Could you check a few things on this drawing? It's one solid part, dimensions in mm from its lowest x, y, z. A direction names the side the tool comes from. Coordinates: 2 decimals unless noted, no trailing zeros. Loops run counter-clockwise (first coordinate to the right, second up) from the corner with the lowest first, then second, coordinate; pieces in that order, holes last. Notation, with made-up numbers: (66.5, 50.25) -> (93.5, 50.25) arc R22 cw to (93.5, 88.25) -> close; hole circle Ø9 at (87, 1.25). An arc over 180 degrees is marked (long way). One line per question, with ' | ' between items.
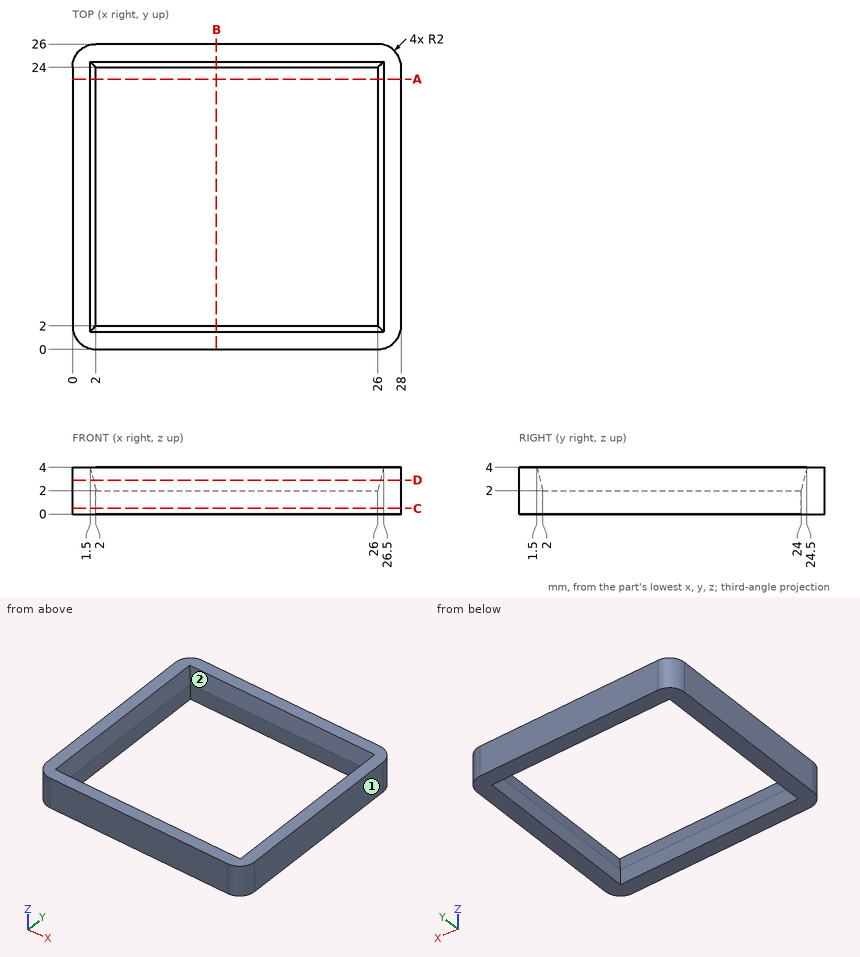
1) If we section it at D-D on z = 2.9: Please give me the cut outline in (x, y) (3 decimals), and give its area (3 significant figures).
Data:
outline: (0, 2) arc R2 ccw to (2, 0) -> (26, 0) arc R2 ccw to (28, 2) -> (28, 24) arc R2 ccw to (26, 26) -> (2, 26) arc R2 ccw to (0, 24) -> close; hole (1.775, 1.775) -> (26.225, 1.775) -> (26.225, 24.225) -> (1.775, 24.225) -> close | area: 176 mm²
2) I need wall thicknesses on line 1 along X through (y, z) = (3.25, 1); line 2 along Y through (x, z) = (10.5, 1.25); line 3 along Y through (x, z) = (6, 2.7) (3 decimals). Which ranges of each line are inside material? Lowest first, please. Write a range as from..to.
Data:
line 1: 0..2, 26..28 | line 2: 0..2, 24..26 | line 3: 0..1.825, 24.175..26
3) If we section it at B-B on x = 12.25: Please give me the cut outline in (y, z).
Data:
outline: (0, 0) -> (2, 0) -> (2, 2) -> (1.5, 4) -> (0, 4) -> close; (24, 0) -> (26, 0) -> (26, 4) -> (24.5, 4) -> (24, 2) -> close
4) If we section it at A-A on y = 23: Please give me the cut outline in (x, z).
Data:
outline: (0, 0) -> (2, 0) -> (2, 2) -> (1.5, 4) -> (0, 4) -> close; (26, 0) -> (28, 0) -> (28, 4) -> (26.5, 4) -> (26, 2) -> close
5) If we section it at C-C on z = 0.5: Please give me the cut outline in (x, y), and give its area (3 significant figures).
Data:
outline: (0, 2) arc R2 ccw to (2, 0) -> (26, 0) arc R2 ccw to (28, 2) -> (28, 24) arc R2 ccw to (26, 26) -> (2, 26) arc R2 ccw to (0, 24) -> close; hole (2, 2) -> (26, 2) -> (26, 24) -> (2, 24) -> close | area: 197 mm²
6) On a 3-axis mill with a long thin cutter (end or side, diameter ignored), from which of +Z, -Z, +X, -X, +Y, -Y can I reach the whole of each face in a straight line? I mean the marked faces 1 and 2. Say none if no direction works.
Data:
face 1: +Z, -Z, +X, +Y, -Y | face 2: +Z
